Input: part model. Units: mm. Frame: model coordinates. Round coordinates to 2 decimals unless told otherwise and drop trailing zeros. Write each loop counter-clockwise with the first axis right and the second up, starting at its lowest first coordinate (ties: lowest second). Pieces come first, ordered by that corner, then holes. Notation, with made-up numbers: (47, 51) - (90, 51) arc R27 cw to (90, 76) - close; hole circle Ø9 at (21, 46). An arc over 180 degrees is marked (long way). One line per item, written item: value. Start each with the question number.
```python
from build123d import *

# Parameters (mm, degrees)
SKETCH1_W           = 857.25
SKETCH1_H           = 450.85
BOSS_EXTRUDE1_DEPTH = 6.35
SKETCH2_R           = 3.175
CUT_EXTRUDE1_DEPTH  = 485.330614095
SKETCH3_R           = 3.175
CUT_EXTRUDE2_DEPTH  = 485.330614095


with BuildPart() as part:
    # Sketch1 → Boss-Extrude1 (new body)
    with BuildSketch(Plane.XY):
        Rectangle(SKETCH1_W, SKETCH1_H)
    extrude(amount=BOSS_EXTRUDE1_DEPTH)

    # Sketch2 → Cut-Extrude1 (cut, through all)
    with BuildSketch(Plane.XY.offset(6.35)):
        with Locations((352.425, -85.725)):
            Circle(SKETCH2_R)
        with Locations((252.425000102, -85.725)):
            Circle(SKETCH2_R)
        with Locations((152.425000204, -85.725)):
            Circle(SKETCH2_R)
        with Locations((52.425000306, -85.725)):
            Circle(SKETCH2_R)
        with Locations((-47.574999592, -85.725)):
            Circle(SKETCH2_R)
        with Locations((276.225, -187.325)):
            Circle(SKETCH2_R)
        with Locations((126.225000026, -187.325)):
            Circle(SKETCH2_R)
        with Locations((-23.774999948, -187.325)):
            Circle(SKETCH2_R)
        with Locations((-173.774999922, -187.325)):
            Circle(SKETCH2_R)
        with Locations((-323.774999896, -187.325)):
            Circle(SKETCH2_R)
        with Locations((276.225, 15.875)):
            Circle(SKETCH2_R)
        with Locations((126.225000026, 15.875)):
            Circle(SKETCH2_R)
        with Locations((-23.774999948, 15.875)):
            Circle(SKETCH2_R)
        with Locations((-173.774999922, 15.875)):
            Circle(SKETCH2_R)
        with Locations((-323.774999896, 15.875)):
            Circle(SKETCH2_R)
        with BuildLine():
            Line((-101.6, -146.05), (101.6, -146.05))
            ThreePointArc((101.6, -146.05), (111.125, -155.575), (101.6, -165.1))
            Line((101.6, -165.1), (-101.6, -165.1))
            ThreePointArc((-101.6, -165.1), (-111.125, -155.575), (-101.6, -146.05))
        make_face()
        with BuildLine():
            Line((193.675, -146.05), (365.125, -146.05))
            ThreePointArc((365.125, -146.05), (374.65, -155.575), (365.125, -165.1))
            Line((365.125, -165.1), (193.675, -165.1))
            ThreePointArc((193.675, -165.1), (184.15, -155.575), (193.675, -146.05))
        make_face()
        with BuildLine():
            Line((365.125, -25.4), (193.675, -25.4))
            ThreePointArc((193.675, -25.4), (184.15, -15.875), (193.675, -6.35))
            Line((193.675, -6.35), (365.125, -6.35))
            ThreePointArc((365.125, -6.35), (374.65, -15.875), (365.125, -25.4))
        make_face()
        with BuildLine():
            Line((101.6, -25.4), (-101.6, -25.4))
            ThreePointArc((-101.6, -25.4), (-111.125, -15.875), (-101.6, -6.35))
            Line((-101.6, -6.35), (101.6, -6.35))
            ThreePointArc((101.6, -6.35), (111.125, -15.875), (101.6, -25.4))
        make_face()
    extrude(amount=-CUT_EXTRUDE1_DEPTH, mode=Mode.SUBTRACT)

    # Sketch3 → Cut-Extrude2 (cut, through all)
    with BuildSketch(Plane.XY.offset(6.35)):
        with Locations((390.525, -100.000000152)):
            Circle(SKETCH3_R)
        with Locations((390.525, 0)):
            Circle(SKETCH3_R)
        with Locations((390.525, 100.000000152)):
            Circle(SKETCH3_R)
    extrude(amount=-CUT_EXTRUDE2_DEPTH, mode=Mode.SUBTRACT)


solid = part.part
```
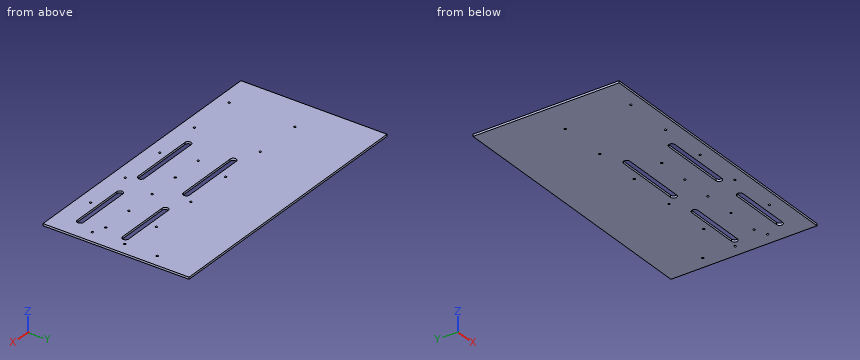
Q1. Material intervals for probe 1 along Y at (x, z) = (358.5, 4.5) (3 decimals); probe 2 along X at (y, z) = (-17.5, 5) (3 decimals); probe 3 along Y at (x, z) = (-21, 1.5) (3 decimals), sorted ascending. Write a range as from..to.
Q2. Cut plane A-A, the plane x = -71. Output: boundary loops of the cut face in (y, z) (3 decimals), and give its area (3 significant figures).
Q3. Contact query for flat-ended pins moving along their axis: pin 1 Ø1.5 at (x, y) = (8.5, 76.5) entering from -Z; pin 2 Ø5.5 at (x, y) = (152.425, -85.725) entering from +Z. Output: stop coordinate, or through.
Q4. Cut plane B-B, the plane z = 2.75. Count the separate pieces of the cut face and the enclosed holes in it, and give its area (3 significant figures).
A:
1. probe 1: y = -225.425..-165.1, -146.05..-25.4, -6.35..225.425
1. probe 2: x = -428.625..-110.985, 110.985..184.29, 374.51..428.625
1. probe 3: y = -225.425..-188.868, -185.782..-165.1, -146.05..-25.4, -6.35..14.332, 17.418..225.425
2. outline: (-225.425, 0) - (-165.1, 0) - (-165.1, 6.35) - (-225.425, 6.35) - close; (-146.05, 0) - (-25.4, 0) - (-25.4, 6.35) - (-146.05, 6.35) - close; (-6.35, 0) - (225.425, 0) - (225.425, 6.35) - (-6.35, 6.35) - close
2. area: 2,620 mm²
3. pin 1: stops at z = 0
3. pin 2: passes through
4. separate pieces: 1
4. enclosed holes: 22
4. area: 371,000 mm²
